The listing builds one solid part. Answer for the finished solid, in the listing's coordinates (mm). A direction names the side the tool comes from. Give positions to 0.01 mm unless a question says otherwise; leave off trailing zeros. Write each loop counter-clockwise with the first axis right and the second up, starting at its lowest first coordinate (ties: lowest second). Pieces come first, ordered by that corner, then holes. Notation, with made-up numbers: (-8.5, 57.5) - (18.5, 57.5) arc R15 cw to (18.5, 81.5) - close; hole circle Ø1 at (76, -23.5). An arc over 180 degrees is marked (long way). Use a Markdown table: item, result. Add a question column.
from build123d import *

# Parameters (mm, degrees)
BOSS_EXTRU_1_DEPTH           = 10
ESQUISSE2_R                  = 7.25
ENL_V_MAT_EXTRU_1_DEPTH      = 11
R_P_TITION_CIRCULAIRE1_COUNT = 7
R_P_TITION_CIRCULAIRE1_ANGLE = 44
R_P_TITION_CIRCULAIRE2_COUNT = 3
R_P_TITION_CIRCULAIRE2_ANGLE = 14.5
ESQUISSE5_W                  = 30
ESQUISSE5_H                  = 30
ENL_V_MAT_EXTRU_2_DEPTH      = 10
CONG_1_R                     = 18
CONG_2_R                     = 3


with BuildPart() as part:
    # Esquisse1 → Boss.-Extru.1 (new body)
    with BuildSketch(Plane.XY):
        with BuildLine():
            Line((75, 0), (-75, 0))
            Line((-75, 0), (-75, 75))
            ThreePointArc((-75, 75), (-5.436050989, 115.40325318), (75, 114.135353054))
            Line((75, 114.135353054), (75, 0))
        make_face()
    extrude(amount=BOSS_EXTRU_1_DEPTH)

    # Esquisse2 → Enlèv. mat.-Extru.1 (cut, through all)
    with BuildSketch(Plane.XY.offset(10)):
        with Locations((28, 104.924979155)):
            Circle(ESQUISSE2_R)
    enl_v_mat_extru_1 = extrude(amount=-ENL_V_MAT_EXTRU_1_DEPTH, mode=Mode.SUBTRACT)

    # Répétition circulaire1: Enlèv. mat.-Extru.1 ×7 about axis
    r_p_tition_circulaire1_axis = Axis((32.5, -30, 0), (0, 0, 1))
    for i in range(1, R_P_TITION_CIRCULAIRE1_COUNT):
        add(enl_v_mat_extru_1.rotate(r_p_tition_circulaire1_axis, i * R_P_TITION_CIRCULAIRE1_ANGLE / (R_P_TITION_CIRCULAIRE1_COUNT - 1)), mode=Mode.SUBTRACT)

    # Répétition circulaire2: Enlèv. mat.-Extru.1 ×3 about axis
    r_p_tition_circulaire2_axis = Axis((32.5, -30, 0), (0, 0, -1))
    for i in range(1, R_P_TITION_CIRCULAIRE2_COUNT):
        add(enl_v_mat_extru_1.rotate(r_p_tition_circulaire2_axis, i * R_P_TITION_CIRCULAIRE2_ANGLE / (R_P_TITION_CIRCULAIRE2_COUNT - 1)), mode=Mode.SUBTRACT)

    # Esquisse5 → Enlèv. mat.-Extru.2 (cut)
    with BuildSketch(Plane.XY.offset(10)):
        with Locations((60, 70)):
            Rectangle(ESQUISSE5_W, ESQUISSE5_H)
    extrude(amount=-ENL_V_MAT_EXTRU_2_DEPTH, mode=Mode.SUBTRACT)

    # Congé1
    cong_1_edges = [part.edges().sort_by_distance(p)[0] for p in [
        (75, 85, 5),
    ]]
    fillet(cong_1_edges, radius=CONG_1_R)

    # Congé2
    cong_2_edges = [part.edges().sort_by_distance(p)[0] for p in [
        (75, 55, 5),
        (45, 55, 5),
        (45, 85, 5),
        (75, 0, 5),
        (-75, 0, 5),
    ]]
    fillet(cong_2_edges, radius=CONG_2_R)


solid = part.part
1. Which of the six approach directions +Z, -Z, +X, -X, +Y, -Y give full straight-line access (tool end or side, diameter ignored) to faces 1 (the cylindrical face through (74.1, 54.14, 4.93)), 2 (the flat face through (-75, 38, 5))?
2. The part is cut by section B-B (z = 7). Count the separate pieces of the cut face and the enclosed holes in it, and give its area (3 significant figures).
3. The part is cut by section A-A (x = 28). Give the vertices of the cut face in (y, z).
4. For a pull along X with two mould halves and no side action, classify faces 3 (the cylindrical face through (45.86, 55.9, 4.93)), 4 (the cylindrical face through (-5.744, 92.144, 5.07)), 5 (the cylindrical face through (-6.54, 115.11, 4.93)) as released by +X, released by -X, zero draft, split by the parting line, or undercut.
5. Consider L1, parallel to X at y = 92, z = 4.25; L2, parallel to X at y = 90, z = 6; L3, parallel to X at y = 105, z = 4.5. Determine where each line is inside the solid, lowest interval first. Write a range as [from, to].
6. Given P1, Ø19, axis at x = -51.68, y = 75.54, coming from the +Z side; P2, Ø1.5, axis at x = -9, z = 6.5, coming from the +Y side; P3, Ø3, axis at y = 74, z = 3.5, coming from the +X side, each flat-ended and moving along its own axis, determine where each tip first touches the part or whether it passes through.
Check values:
| question | item | result |
|---|---|---|
| 1 | face 1 | +Z, -Z, +X |
| 1 | face 2 | +Z, -Z, -X, +Y, -Y |
| 2 | separate pieces | 1 |
| 2 | enclosed holes | 9 |
| 2 | area | 14,000 mm2 |
| 3 | outline | (0, 0) - (97.67, 0) - (97.67, 10) - (0, 10) - close; (112.17, 0) - (120.2, 0) - (120.2, 10) - (112.17, 10) - close |
| 4 | face 3 | released by +X |
| 4 | face 4 | undercut |
| 4 | face 5 | split by the parting line |
| 5 | L1 | x = [-55.23, -40.57], [-34.48, -29.33], [-15.11, 71.25] |
| 5 | L2 | x = [-57.95, -43.14], [-31.9, -28.61], [-15.82, 69.45] |
| 5 | L3 | x = [-33.5, -10.61], [-1.42, 3.78], [17.85, 20.75], [35.25, 37.84], [52.29, 55.44], [68.41, 75] |
| 6 | P1 | stops at z = 10 |
| 6 | P2 | stops at y = 114.64 |
| 6 | P3 | stops at x = 45 |
